from build123d import *

# Parameters (mm, degrees)
SKETCH1_R                = 1.55
BOSS_EXTRUDE1_DEPTH      = 35
BOSS_EXTRUDE1_DEPTH_BACK = 35


with BuildPart() as part:
    # Sketch1 → Boss-Extrude1 (new body, two sides)
    with BuildSketch(Plane(origin=(0, 0, 0), x_dir=(0, 0, -1), z_dir=(1, 0, 0))) as boss_extrude1_sk:
        Circle(SKETCH1_R)
    extrude(amount=BOSS_EXTRUDE1_DEPTH)
    extrude(boss_extrude1_sk.sketch, amount=-BOSS_EXTRUDE1_DEPTH_BACK)

    # Sketch3 → M2x0.25 Tapped Hole1 (revolve, cut)
    with BuildSketch(Plane(origin=(35, 0, 0), x_dir=(0, 0, -1), z_dir=(0, 1, 0))):
        Polygon((0, 0), (0, 10.525753042), (0.875, 10), (0.875, 0), align=None)
    m2x0_25_tapped_hole1 = revolve(axis=Axis((41.35, 0, 0), (-1, 0, 0)), mode=Mode.SUBTRACT)

    # Mirror1: M2x0.25 Tapped Hole1 across plane
    add(m2x0_25_tapped_hole1.mirror(Plane(origin=(0, 0, 0), x_dir=(0, 0, 1), z_dir=(1, 0, 0))), mode=Mode.SUBTRACT)


solid = part.part
Build history of the part. All positions in model axes, mm. A direction names the side the tool comes from. Give positions to 0.01 mm unless a question says otherwise; leave off trailing zeros. Loops run counter-clockwise (first coordinate to the right, second up) from the corner with the lowest first, then second, coordinate; pieces in that order, holes last. Notation, with made-up numbers: (-32.5, 57.5) - (-10.5, 57.5) arc R21 ccw to (-10.5, 67.5) - close; hole circle Ø3 at (4, 54.5). An arc over 180 degrees is marked (long way). Write item = value, one per line. Start each with the question number.
1) Tool access for faces 5 (the conical face through (-24.566, 0.148, 0.033)), 6 (the cylindrical face through (30.07, 0.335, -0.808)): list every direction of +Z, -Z, +X, -X, +Y, -Y with a clear straight run to the whole face (end or side of a thin tool).
2) Pull direction Z, two halves, no side cores. Call faces 1 (the flat face through (-35, -1, -0.3)), 2 (the cylindrical face through (0.49, -1.375, -0.715)), 3 (the cylindrical face through (-30.07, 0.335, -0.808)), 4 (the conical face through (24.566, 0.148, 0.033)): +Z half, -Z half, draft (parallel to the pull), parting line (faces both ways), or undercut.
3) Probe probe 1 along Y at (x, z) = (30.25, 0) (3 decimals); probe 2 along Y at (x, z) = (-13, 0.15); probe 3 along Z at (x, y) = (-13, 1). List the from-to ranges inside material, lowest first. Write a range as from..to.
4) Drop flat-ended pins along their axis: pin 1 Ø1.5 at (x, z) = (18, 1) entering from +Y; pin 2 Ø1.4 at (y, z) = (0, 0) entering from -X. Give the stop position or say it passes through.
5) Band-saw the part on B-B on x = 21.5. Give the cut face in (y, z).
6) Band-saw the part on A-A on x = -29. Give the cut face in (y, z) (3 decimals), plus the area to 3 significant figures.
Final values:
q1.face_5 = -X
q1.face_6 = +X
q2.face_1 = draft
q2.face_2 = parting line
q2.face_3 = undercut
q2.face_4 = undercut
q3.probe_1 = -1.55..-0.875, 0.875..1.55
q3.probe_2 = -1.54..1.54
q3.probe_3 = -1.18..1.18
q4.pin_1 = 1.53
q4.pin_2 = -24.89
q5.outline = circle Ø3.1 at (0, 0)
q6.outline = circle Ø3.1 at (0, 0); hole circle Ø1.75 at (0, 0)
q6.area = 5.14 mm²
